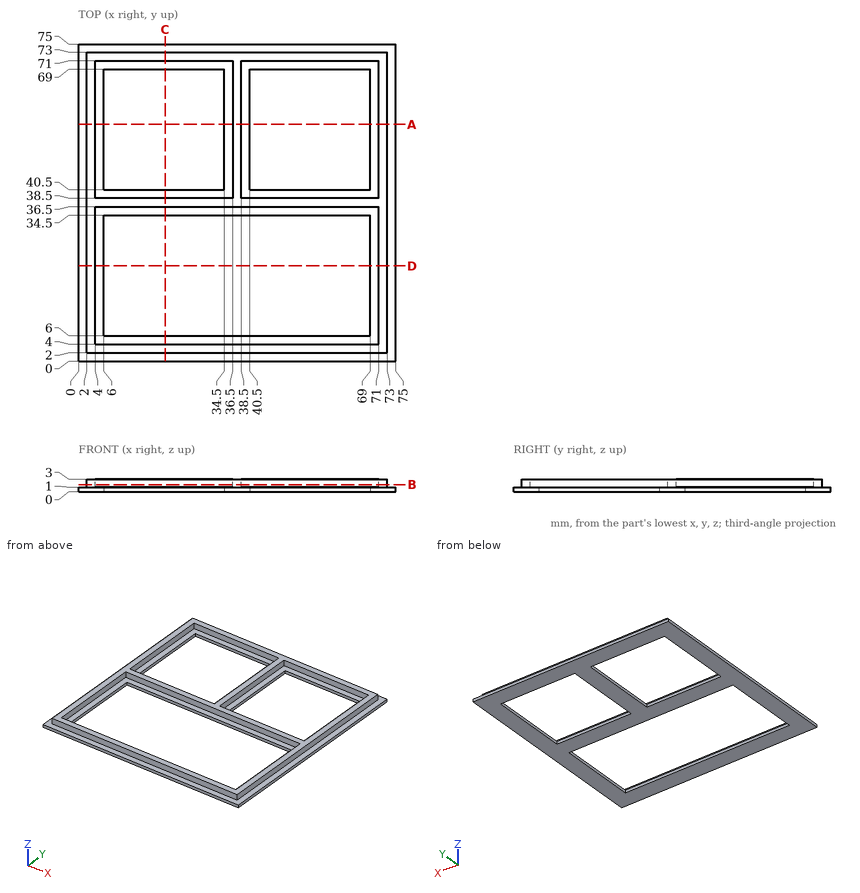
Answer from the drawing. Dimensions are ordinates in mm from the lowest x, y and z of the part. Give positions to 0.01 mm unless a question says otherwise; leave off trailing zeros. Order: outer loops, then holes, each group sorted by start corner. A loop starts at its lowest first (then second) coordinate and runs counter-clockwise, first axis right, second up. Notation, with made-up numbers: (3, 60.25) -> (11, 60.25) arc R6 cw to (11, 69.25) -> close; hole circle Ø5 at (49.25, -25.75). An arc over 180 degrees is marked (long way). Answer as a JSON object with one key per item and string values. Group by question number.
1. Section D-D on y = 22.5 is taken. Determine the outline of the cut face in (x, z), plus the area to 3 significant figures.
2. Consider line 1 along Y through (x, z) = (33, 2.4); line 2 along X through (y, z) = (59.5, 0.35). Determine where each line is inside the solid, lowest interval first. Write a range as [from, to].
3. Section A-A on y = 56 is taken. Determine the outline of the cut face in (x, z).
4. Flat-ended cylindrical pins translate along their axes: pin 1 Ø0.6 at (y, z) = (49.5, 1.5) entering from +X; pin 2 Ø1.6 at (y, z) = (57.5, 2.5) entering from -X; pin 3 Ø0.6 at (x, z) = (61.5, 2.5) entering from +Y. Find the tip coordinate at first contact, or state that the pin passes through.
5. Section B-B on z = 1.65 is taken. Determine the outline of the cut face in (x, y), plus the area to 3 significant figures.
Result sheet:
{
 "1": {"outline": "(0, 0) -> (6, 0) -> (6, 1) -> (4, 1) -> (4, 3) -> (2, 3) -> (2, 1) -> (0, 1) -> close; (69, 0) -> (75, 0) -> (75, 1) -> (73, 1) -> (73, 3) -> (71, 3) -> (71, 1) -> (69, 1) -> close", "area": "20.0 mm^2"},
 "2": {"line 1": "y = [2, 4], [36.5, 38.5], [71, 73]", "line 2": "x = [0, 6], [34.5, 40.5], [69, 75]"},
 "3": {"outline": "(0, 0) -> (6, 0) -> (6, 1) -> (4, 1) -> (4, 3) -> (2, 3) -> (2, 1) -> (0, 1) -> close; (34.5, 0) -> (40.5, 0) -> (40.5, 1) -> (38.5, 1) -> (38.5, 3) -> (36.5, 3) -> (36.5, 1) -> (34.5, 1) -> close; (69, 0) -> (75, 0) -> (75, 1) -> (73, 1) -> (73, 3) -> (71, 3) -> (71, 1) -> (69, 1) -> close"},
 "4": {"pin 1": "stops at x = 73", "pin 2": "stops at x = 2", "pin 3": "stops at y = 73"},
 "5": {"outline": "(2, 2) -> (73, 2) -> (73, 73) -> (2, 73) -> close; hole (4, 4) -> (71, 4) -> (71, 36.5) -> (4, 36.5) -> close; hole (4, 38.5) -> (36.5, 38.5) -> (36.5, 71) -> (4, 71) -> close; hole (38.5, 38.5) -> (71, 38.5) -> (71, 71) -> (38.5, 71) -> close", "area": "751 mm^2"}
}
